Verification items for the finished model (mm, model axes). A direction names the side the tool comes from. Round coordinates to 2 decimals unless told otherwise and drop trailing zeros. Order: outer loops, then holes, each group sorted by start corner. A loop starts at its lowest first (then second) coordinate and runs counter-clockwise, first axis right, second up. Notation, with made-up numbers: (-1.5, 88) -> (42.5, 88) arc R22 ccw to (42.5, 105) -> close; hole circle Ø3 at (63, 69.25). An arc over 180 degrees is marked (long way). Return JSON: item names as keys, results as strings. Group by question number.
1) Depth check by flat-ended pin: pin 1 (4 mm diameter, centred on y = -6, z = 41.5, fed in from -X); pin 2 (1 mm diameter, centred on x = -20.5, z = 21.5, fed in from -Y); pin 3 (1.5 mm diameter, centred on x = 29.5, y = -32.5, fed in from +Z). Enter the tip coordinate at first touch or a pass-through.
2) Section check D-D on z = 32.5. Enter the section's corners in (x, y).
3) Tool access check on faces 4 (the flat face through (22.22, -16.49, 31.66)), 5 (the flat face through (-8.818, -26.228, 31.661)), 6 (the flat face through (-27.669, 0, 32)). Record the directions out of +Z, -Z, +X, -X, +Y, -Y that give a thin tool (end or side, any length) a straight path to the whole face; none if there is none.
4) Scan lines: L1, parallel to Z at x = -5, y = -36.5; L2, parallel to Y at x = -8, z = 34; L3, parallel to X at y = 7.5, z = 4. Record each from-to range of solid material in increasing order.
5) Section check A-A on z = 43.5. Enter the section's corners in (x, y), plus the area to 3 significant figures.
6) Section check B-B on y = 11.5. Enter the section's corners in (x, z), plus the area to 3 significant figures.
7) Draft check along Y on faces 1 (the flat face through (22.55, 16.036, 31.661)), 2 (the flat face through (-11.33, -33.71, 18.96)), 3 (the flat face through (-3.58, -11.413, 25.044)). Enter one of: pulls with the +Y half, pulls with the -Y half, needs draft (parallel to the pull), parting line crosses it, or undercut.
8) Section check C-C on x = 40. Enter the section's corners in (y, z).
```python
from build123d import *

# Parameters (mm, degrees)
F1_DEPTH = 12.7
F2_DEPTH = 25.4
F3_DEPTH = 38.1
F4_DEPTH = 50.8


with BuildPart() as f1:
    # F0 (on Top) → F1 (new body)
    with BuildSketch(Plane.XY):
        Polygon((-42.968333, 31.218321), (-42.968333, -31.218321), (16.412443, -50.512305), (53.11178, 0), (16.412443, 50.512305), align=None)
        Polygon((13.582712, -41.803288), (-35.560001, -25.835853), (-35.560001, 25.835853), (13.582712, 41.803288), (43.954578, 0), align=None, mode=Mode.SUBTRACT)
    extrude(amount=F1_DEPTH)

    # F0 (on Top) → F2 (join)
    with BuildSketch(Plane.XY):
        Polygon((-35.560001, 25.835853), (-35.560001, -25.835853), (13.582712, -41.803288), (43.954578, 0), (13.582712, 41.803288), align=None)
        Polygon((10.568597, 32.526797), (34.200698, 0), (10.568597, -32.526797), (-27.668946, -20.102666), (-27.668946, 20.102666), align=None, mode=Mode.SUBTRACT)
    extrude(amount=F2_DEPTH)

    # F0 (on Top) → F3 (join)
    with BuildSketch(Plane.XY):
        Polygon((10.568597, -32.526797), (34.200698, 0), (10.568597, 32.526797), (-27.668946, 20.102666), (-27.668946, -20.102666), align=None)
        Polygon((7.614722, 23.435704), (24.641757, 0), (7.614722, -23.435704), (-19.9356, -14.484062), (-19.9356, 14.484062), align=None, mode=Mode.SUBTRACT)
    extrude(amount=F3_DEPTH)

    # F0 (on Top) → F4 (join)
    with BuildSketch(Plane.XY):
        Polygon((7.614722, -23.435704), (24.641757, 0), (7.614722, 23.435704), (-19.9356, 14.484062), (-19.9356, -14.484062), align=None)
        Polygon((4.568539, 14.060516), (14.784101, 0), (4.568539, -14.060516), (-11.960589, -8.689877), (-11.960589, 8.689877), align=None, mode=Mode.SUBTRACT)
    extrude(amount=F4_DEPTH)


solid = f1.part
```
Check result:
{
 "1": {"pin 1": "x = -19.94", "pin 2": "y = -30.89", "pin 3": "z = 12.7"},
 "2": {"outline": "(-27.67, -20.1) -> (10.57, -32.53) -> (34.2, 0) -> (10.57, 32.53) -> (-27.67, 20.1) -> close; hole (-11.96, -8.69) -> (4.57, -14.06) -> (14.78, 0) -> (4.57, 14.06) -> (-11.96, 8.69) -> close"},
 "3": {"face 4": "+Z, +X, -Y", "face 5": "+Z, -X, -Y", "face 6": "+Z, -X, +Y, -Y"},
 "4": {"L1": "0 to 12.7", "L2": "-26.49 to -9.98, 9.98 to 26.49", "L3": "-42.97 to -11.96, 9.34 to 47.66"},
 "5": {"outline": "(-19.94, -14.48) -> (7.61, -23.44) -> (24.64, 0) -> (7.61, 23.44) -> (-19.94, 14.48) -> close; hole (-11.96, -8.69) -> (4.57, -14.06) -> (14.78, 0) -> (4.57, 14.06) -> (-11.96, 8.69) -> close", "area": "924 mm^2"},
 "6": {"outline": "(-42.97, 0) -> (-3.31, 0) -> (-3.31, 50.8) -> (-19.94, 50.8) -> (-19.94, 38.1) -> (-27.67, 38.1) -> (-27.67, 25.4) -> (-35.56, 25.4) -> (-35.56, 12.7) -> (-42.97, 12.7) -> close; (6.43, 0) -> (44.76, 0) -> (44.76, 12.7) -> (35.6, 12.7) -> (35.6, 25.4) -> (25.85, 25.4) -> (25.85, 38.1) -> (16.29, 38.1) -> (16.29, 50.8) -> (6.43, 50.8) -> close", "area": "2,660 mm^2"},
 "7": {"face 1": "pulls with the +Y half", "face 2": "pulls with the -Y half", "face 3": "undercut"},
 "8": {"outline": "(-18.05, 0) -> (18.05, 0) -> (18.05, 12.7) -> (5.44, 12.7) -> (5.44, 25.4) -> (-5.44, 25.4) -> (-5.44, 12.7) -> (-18.05, 12.7) -> close"}
}
